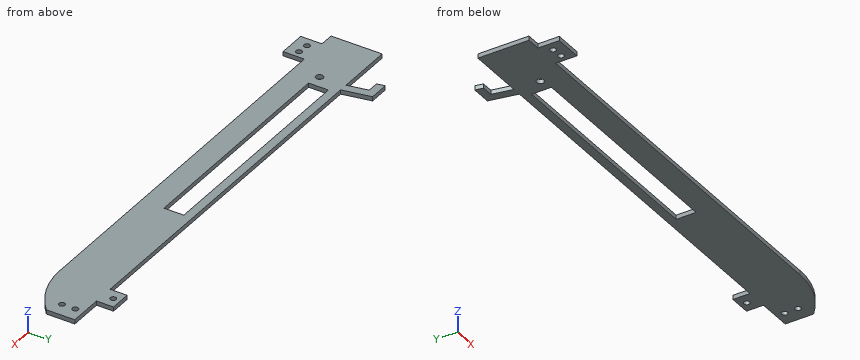
Autodesk Inventor part; units mm, degrees
ref_plane "YZ Plane" through (0, 0, 0) normal (1, 0, 0) x (0, 1, 0)
ref_plane "XZ Plane" through (0, 0, 0) normal (0, 1, 0) x (-1, 0, 0)
ref_plane "XY Plane" through (0, 0, 0) normal (0, 0, 1) x (1, 0, 0)
sketch "Sketch1" plane through (0, 0, 0) normal (0, 0, 1) x (1, 0, 0)
  line L0 (0, 0) -> (300, 0)
  line L1 (300, 0) -> (300, 16)
  line L2 (300, 16) -> (0, 16)
  line L3 (0, 16) -> (0, 0)
  line L4 (0, 0) -> (22.0483, 0)
  line L5 (10, 0) -> (29.5, 0)
  line L6 (29.5, 0) -> (29.5, -15)
  line L7 (29.5, -15) -> (10, -15)
  line L8 (10, -15) -> (10, 0)
  point P0 (0, 8)
  dimension "d2" = 19.5
  dimension "d3" = 15
  dimension "d4" = 10
  dimension "d5" = 16
  dimension "d8" = 300
extrude "Extrusion1" add sketch "Sketch1" along normal blind 3
sketch "Sketch2" plane through (0, 0, 3) normal (0, 0, 1) x (1, 0, 0)
  line L0 (0, 16) -> (0, 0)
  line L1 (0, 16) -> (0, 36)
  line L2 (300, 0) -> (300, 16)
  line L3 (340, 16) -> (340, 36)
  line L4 (340, 36) -> (0, 36)
  line L5 (300, 16) -> (0, 16)
  line L6 (50, 16) -> (50, 30)
  line L7 (50, 30) -> (210, 30)
  line L8 (210, 30) -> (210, 16)
  line L9 (40, 36) -> (36, 56)
  line L10 (36, 56) -> (42, 56)
  line L11 (42, 56) -> (46, 36)
  circle A0 centre (330, 30) radius 2.1
  circle A1 centre (330, 20.6) radius 2.1
  line L12 (340, 16) -> (300, 16)
  line L13 (301, 36) -> (316, 36)
  line L14 (316, 36) -> (316, 48)
  line L15 (316, 48) -> (301, 48)
  line L16 (301, 48) -> (301, 36)
  circle A2 centre (308.5, 43) radius 2.075
  line L17 (36, 56) -> (28, 56)
  line L18 (28, 56) -> (29.1, 50.5)
  line L19 (29.1, 50.5) -> (37.1, 50.5)
  point P0 (308.5, 48)
  point P1 (316, 36)
  dimension "d44" = 20
  dimension "d45" = 160
  dimension "d46" = 50
  dimension "d47" = 14
  dimension "d48" = 20
  dimension "d49" = 6
  dimension "d50" = 4
  dimension "d51" = 40
  dimension "d83" = 4.2
  dimension "d84" = 4.2
  dimension "d85" = 6
  dimension "d86" = 9.4
  dimension "d87" = 10
  dimension "d99" = 40
  dimension "d107" = 7
  dimension "d108" = 15
  dimension "d109" = 12
  dimension "d110" = 24
  dimension "d111" = 4.15
  dimension "d112" = 8
  dimension "d114" = 5.5
extrude "Extrusion2" add sketch "Sketch2" against normal blind 3 contours L1 L4 L3 L12 L5 L8 L7 L6 | L9 L10 L11 L4 | L19 L18 L17 L9 | L16 L15 L14 L4
sketch "Sketch3" plane through (0, 0, 3) normal (0, 0, 1) x (1, 0, 0)
  circle A0 centre (16.5, -6.5) radius 2.1
  circle A1 centre (24.5, -7) radius 2.1
  line L0 (29.5, 0) -> (300, 0)
  line L1 (29.5, -15) -> (29.5, 0)
  point P0 (0, 0)
  dimension "d75" = 4.2
  dimension "d76" = 6.5
  dimension "d77" = 4.2
  dimension "d78" = 7
  dimension "d79" = 5
  dimension "d80" = 8
extrude "Extrusion3" cut sketch "Sketch3" against normal blind 3
sketch "Sketch4" plane through (0, 0, 3) normal (0, 0, 1) x (1, 0, 0)
  line L0 (29.5, 0) -> (300, 0)
  circle A0 centre (41, 18) radius 2.6
  line L1 (340, 36) -> (46, 36)
  line L2 (38.4, 28.1) -> (43.6, 28.1)
  line L3 (43.6, 28.1) -> (43.6, 7.9)
  line L4 (43.6, 7.9) -> (38.4, 7.9)
  line L5 (38.4, 7.9) -> (38.4, 28.1)
  line L6 (38.4, 28.1) -> (43.6, 7.9) construction
  line L7 (43.6, 28.1) -> (38.4, 7.9) construction
  point P0 (0, 0)
  point P1 (43.6, 18)
  point P2 (38.4, 18)
  dimension "d95" = 18
  dimension "d96" = 5.2
  dimension "d100" = 5
  dimension "d101" = 20.2
extrude "Extrusion4" cut sketch "Sketch4" against normal blind 3 contours A0
sketch "Sketch5" plane through (0, 0, 3) normal (0, 0, 1) x (1, 0, 0)
  line L0 (29.5, 0) -> (300, 0)
  line L1 (340, 36) -> (340, 16)
  arc A0 (300, 0) -> (340, 16) centre (300, 58) ccw
  line L2 (300, 0) -> (300, 16)
  line L3 (300, 0) -> (300, 16)
  line L4 (300, 16) -> (340, 16)
  point P0 (0, 0)
extrude "Extrusion5" add sketch "Sketch5" against normal blind 3
properties part number "Middle_bar"
For this review, take the finished solid that the model builds, in its own axes (mm). Round coordinates to 2 decimals unless told otherwise and drop trailing zeros. Write each loop counter-clockwise with the first axis right and the second up, starting at its lowest first coordinate (ties: lowest second). Pieces come first, ordered by that corner, then holes. Notation, with made-up numbers: M -26,70.25 L 11,70.25 A10 cw 11,76.25 Z; hole C -28,45 d9. An arc over 180 degrees is marked long. Write item = value, one per line. Start each with the question number.
(1) We need section C-C (x = 164.5). Give the boundary of the cut face in (y, z), then the cut area to 3 significant figures.
(2) For line 1 along X through (y, z) = (18, 2.35); line 2 along Y through (x, z) = (24.5, 0.8); line 3 along X through (y, z) = (22, 0.6), list the stretches that pass through material, from the lowest coordinate up.
(3) We need section B-B (z = 1.8). Give the number of separate pieces and of enclosed holes in the cut face, then the cut area to 3 significant figures.
(4) Clearance check with flat-ended pins moving along their axes: pin 1 Ø1.5 at (x, z) = (4, 2) entering from -Y; pin 2 Ø0.9 at (x, z) = (328, 2) entering from +Y; pin 3 Ø0.9 at (y, z) = (41, 1) entering from +X. State where each tip first meets the part, or that it passes through.
(5) We need section A-A (x = 33). Give the boundary of the cut face in (y, z), then the cut area to 4 significant figures.
(6) We need section D-D (x = 291.5). Give the boundary of the cut face in (y, z), then the cut area to 3 significant figures.
Results found:
q1.outline = M 0,0 L 16,0 L 16,3 L 0,3 Z; M 30,0 L 36,0 L 36,3 L 30,3 Z
q1.area = 66.0 mm²
q2.line_1 = 0 to 38.4, 43.6 to 50, 210 to 340
q2.line_2 = -15 to -9.1, -4.9 to 36
q2.line_3 = 0 to 50, 210 to 328.43, 331.57 to 340
q3.separate_pieces = 1
q3.enclosed_holes = 7
q3.area = 10,300 mm²
q4.pin_1 = 0
q4.pin_2 = 36
q4.pin_3 = 316
q5.outline = M 0,0 L 36,0 L 36,3 L 0,3 Z; M 50.5,0 L 56,0 L 56,3 L 50.5,3 Z
q5.area = 124.5 mm²
q6.outline = M 0,0 L 36,0 L 36,3 L 0,3 Z
q6.area = 108 mm²
